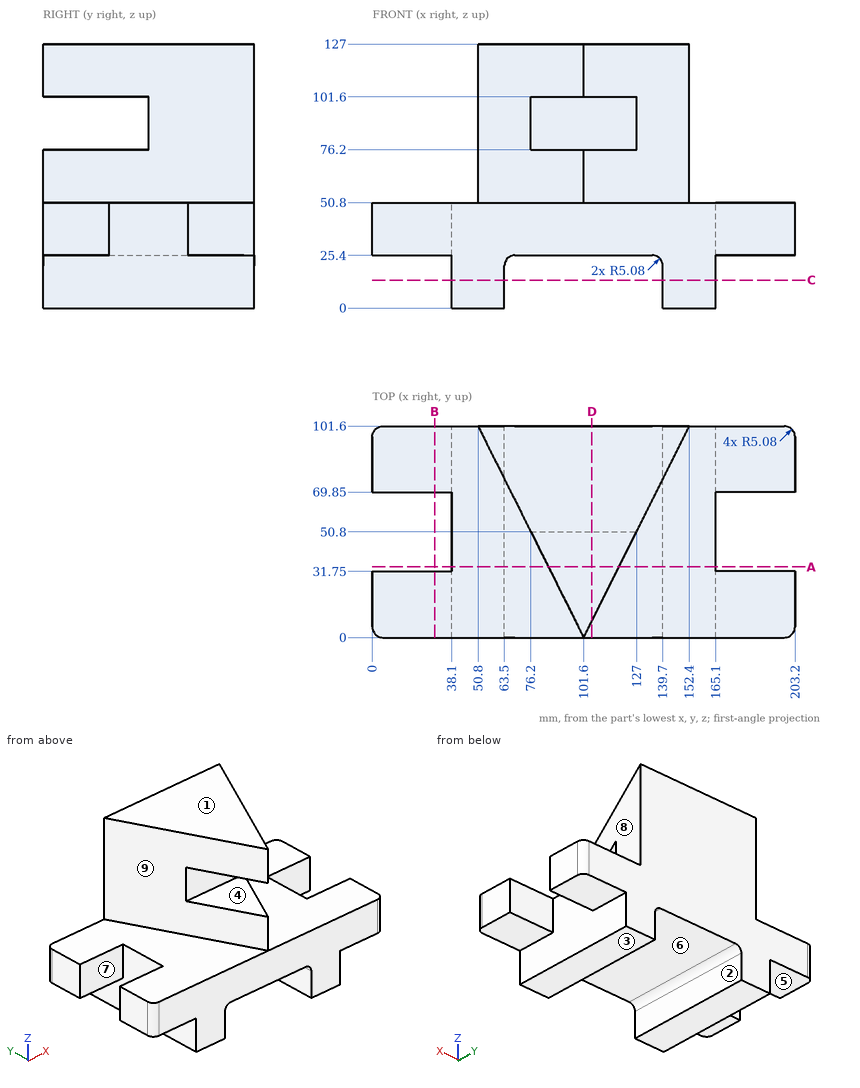
Answer from the drawing. Dimensions are ordinates in mm from the lowest x, y and z of the part. A direction names the side the tool comes from. Give positions to 0.01 mm unless a question says otherwise; leave off trailing zeros. Order: outer loops, then holes, each group sorted by start corner. A loop starts at its lowest first (then second) coordinate and runs counter-clockwise, first axis right, second up. Notation, with made-up numbers: (-18.75, 60) - (35.25, 60) arc R26 cw to (35.25, 86) - close; hole circle Ø6 at (-5, 23). An arc over 180 degrees is marked (long way). One line per item, written item: value. Start each with the question number.
1) A cutting plane is placed at B-B on x = 30. Give the vertices of the cut face in (y, z).
2) A cutting plane is placed at D-D on x = 105.5. Give the vertices of the cut face in (y, z).
3) A tool of negligible diameter and unlimited length cuts with its end or side. For the marked faces 5, 6, 7, 8 and 9, from which of +Z, -Z, +X, -X, +Y, -Y can it reach the whole face along a straight path? Write none if from no direction.
4) A cutting plane is placed at C-C on z = 13.5. Give the vertices of the cut face in (x, y).
5) Find the intervals of material crossed by L1, parallel to Z at x = 113, y = 42; L2, parallel to Z at x = 190, y = 7; L3, parallel to Z at x = 94.5, y = 90, in increasing order.
6) The mould has two halves that part along Z. Classify the marked faces 1, 2, 3 and 4: released by +Z, released by -Z, zero draft, split by the parting line, or undercut.
7) Given pin 1 Ø9.5 at (x, y) = (190, 81.5) entering from -Z; pin 2 Ø10 at (y, z) = (52, 10) entering from -X; pin 3 Ø8 at (x, z) = (155, 83) entering from -Y, each flat-ended and moving along its own axis, determine where each tip first touches the part or whether it passes through.
8) A cutting plane is placed at A-A on y = 34. Give the vertices of the cut face in (x, z), then the cut area to 3 significant figures.
Answer sheet:
1. outline: (0, 25.4) - (31.75, 25.4) - (31.75, 50.8) - (0, 50.8) - close; (69.85, 25.4) - (101.6, 25.4) - (101.6, 50.8) - (69.85, 50.8) - close
2. outline: (0, 25.4) - (101.6, 25.4) - (101.6, 127) - (7.8, 127) - (7.8, 101.6) - (50.8, 101.6) - (50.8, 76.2) - (7.8, 76.2) - (7.8, 50.8) - (0, 50.8) - close
3. face 5: -Z, -X, +Y, -Y
3. face 6: -Z, +Y, -Y
3. face 7: +Z, -Z, -X
3. face 8: +Z, +X, -Y
3. face 9: +Z, -X, -Y
4. outline: (38.1, 0) - (63.5, 0) - (63.5, 101.6) - (38.1, 101.6) - close; (139.7, 0) - (165.1, 0) - (165.1, 101.6) - (139.7, 101.6) - close
5. L1: z = 25.4 to 76.2, 101.6 to 127
5. L2: z = 25.4 to 50.8
5. L3: z = 25.4 to 127
6. face 1: released by +Z
6. face 2: zero draft
6. face 3: released by -Z
6. face 4: undercut
7. pin 1: stops at z = 25.4
7. pin 2: stops at x = 38.1
7. pin 3: stops at y = 98.8
8. outline: (38.1, 0) - (63.5, 0) - (63.5, 20.32) arc R5.08 cw to (68.58, 25.4) - (134.62, 25.4) arc R5.08 cw to (139.7, 20.32) - (139.7, 0) - (165.1, 0) - (165.1, 50.8) - (118.6, 50.8) - (118.6, 76.2) - (84.6, 76.2) - (84.6, 50.8) - (38.1, 50.8) - close; (84.6, 101.6) - (118.6, 101.6) - (118.6, 127) - (84.6, 127) - close
8. area: 6,250 mm2
